from build123d import *

# Parameters (mm, degrees)
EXTRUDE_THIN1_START = -15.875
EXTRUDE_THIN1_DEPTH = 31.75
SKETCH4_R           = 2.0828
EXTRUDE3_DEPTH      = 56.149155941
CIRPATTERN1_COUNT   = 2


# Read off the part's stored shape, not the designer's step: Extrude-Thin1
with BuildPart() as part:
    # Extrude-Thin1 outline → Extrude-Thin1 (new body)
    with BuildSketch(Plane(origin=(0, 0, 0), x_dir=(1, 0, 0), z_dir=(0, 1, 0)).offset(EXTRUDE_THIN1_START)):
        with BuildLine():
            Line((2.286, -1.524), (38.1, -1.524))
            Line((38.1, -1.524), (38.1, 0))
            Line((38.1, 0), (2.286, 0))
            ThreePointArc((2.286, 0), (0.669553898, -0.669553898), (0, -2.286))
            Line((0, -2.286), (0, -38.1))
            Line((0, -38.1), (1.524, -38.1))
            Line((1.524, -38.1), (1.524, -2.286))
            ThreePointArc((1.524, -2.286), (1.747184633, -1.747184633), (2.286, -1.524))
        make_face()
    extrude(amount=EXTRUDE_THIN1_DEPTH)

    # Sketch4 → Extrude3 (cut, through all)
    with BuildSketch(Plane(origin=(1.524, 0, 0), x_dir=(0, 0, -1), z_dir=(1, 0, 0))):
        with Locations((-31.75, 60.325)):
            Circle(SKETCH4_R)
        with Locations((-9.525, 41.275)):
            Circle(SKETCH4_R)
        with Locations((-9.525, -9.525)):
            Circle(SKETCH4_R)
        with Locations((-31.75, 9.525)):
            Circle(SKETCH4_R)
    extrude3 = extrude(amount=-EXTRUDE3_DEPTH, mode=Mode.SUBTRACT)

    # CirPattern1: Extrude3 ×2 about axis
    cirpattern1_axis = Axis((0, 0, 0), (0.7071067811865464, 0, 0.7071067811865487))
    for i in range(1, CIRPATTERN1_COUNT):
        add(extrude3.rotate(cirpattern1_axis, i * 360 / CIRPATTERN1_COUNT), mode=Mode.SUBTRACT)


solid = part.part
Verification items for the finished model (mm, model axes). A direction names the side the tool comes from. Give positions to 0.01 mm unless a question says otherwise; leave off trailing zeros. Write each loop counter-clockwise with the first axis right and the second up, starting at its lowest first coordinate (ties: lowest second). Pieces come first, ordered by that corner, then holes. Notation, with made-up numbers: (14.5, 66) -> (41.5, 66) arc R28 cw to (41.5, 92) -> close; hole circle Ø10 at (37, -18.5). An arc over 180 degrees is marked (long way). Use CSV: the item, a comma, the result in double quotes.
(1) Go/stop test with flat-tipped pins: pin 1 (3.5 mm diameter, centred on y = 9.525, z = 31.75, fed in from -X) (3 decimals); pin 2 (9.5 mm diameter, centred on x = 13, y = 1.5, fed in from +Z); pin 3 (5 mm diameter, centred on y = -9.525, z = 9.525, fed in from +X). Record where each tip stops, or that it passes through.
Derived:
pin 1,"passes through"
pin 2,"stops at z = 1.52"
pin 3,"stops at x = 1.52"
(2) Sectioned sample at B-B (x = 31.75). Record the cut outline in (y, z) (3 decimals), plus the area to 3 significant figures.
Derived:
outline,"(-15.875, 0) -> (-11.608, 0) -> (-11.608, 1.524) -> (-15.875, 1.524) -> close; (-7.442, 0) -> (15.875, 0) -> (15.875, 1.524) -> (-7.442, 1.524) -> close"
area,"42.0 mm^2"
(3) Sectioned sample at C-C (y = -11). Record the cut outline in (x, z).
Derived:
outline,"(0, 2.29) arc R2.29 ccw to (2.29, 0) -> (30.28, 0) -> (30.28, 1.52) -> (2.29, 1.52) arc R0.76 cw to (1.52, 2.29) -> (1.52, 8.05) -> (0, 8.05) -> close; (0, 11) -> (1.52, 11) -> (1.52, 38.1) -> (0, 38.1) -> close; (33.22, 0) -> (38.1, 0) -> (38.1, 1.52) -> (33.22, 1.52) -> close"
(4) Release check for a two-part mould opening along Y. For faces 3 (the flat face through (1.524, 0, 20)), 4 (the cylindrical face through (33.83, -9.62, 0.77)), 5 (the cylindrical face through (0.77, -7.46, 9.8)), 6 (the flat face through (1, 15.875, 10)) record: +Y half, -Y half, draft (parallel to the pull), parting line (faces both ways), or undercut.
Derived:
face 3,"draft"
face 4,"undercut"
face 5,"undercut"
face 6,"+Y half"
(5) Material ranges on L1, parallel to X at y = -4, z = 20; L2, parallel to Y at x = 31, z = 1 (3 decimals), recorded low to high.
Derived:
L1,"x = 0 to 1.52"
L2,"y = -15.875 to -11.468, -7.582 to 15.875"
(6) Set-up check for faces 1 (the cylindrical face through (0.69, -0.22, 0.65)), 2 (the flat face through (20, 0, 1.524)): record each of +Z, -Z, +X, -X, +Y, -Y from which the full face is reachable in a straight line by a thin tool's end or side.
Derived:
face 1,"-Z, -X, +Y, -Y"
face 2,"+Z, +X, +Y, -Y"
(7) Sectioned sample at D-D (y = 6). Record the cut outline in (x, z).
Derived:
outline,"(0, 2.29) arc R2.29 ccw to (2.29, 0) -> (38.1, 0) -> (38.1, 1.52) -> (2.29, 1.52) arc R0.76 cw to (1.52, 2.29) -> (1.52, 38.1) -> (0, 38.1) -> close"
(8) Sectioned sample at A-A (z = 31.75). Record the cut outline in (x, y) (3 decimals).
Derived:
outline,"(0, -15.875) -> (1.524, -15.875) -> (1.524, 7.442) -> (0, 7.442) -> close; (0, 11.608) -> (1.524, 11.608) -> (1.524, 15.875) -> (0, 15.875) -> close"
